```python
from build123d import *

# Parameters (mm, degrees)
SKETCH1_W           = 120
SKETCH1_H           = 90
BOSS_EXTRUDE1_DEPTH = 3
SKETCH2_W           = 4
SKETCH2_H           = 1.5
BOSS_EXTRUDE2_DEPTH = 15


with BuildPart() as part:
    # Sketch1 → Boss-Extrude1 (new body)
    with BuildSketch(Plane(origin=(0, 0, 0), x_dir=(0, 1, 0), z_dir=(0, 0, 1))):
        with Locations((-60, 45)):
            Rectangle(SKETCH1_W, SKETCH1_H)
    extrude(amount=BOSS_EXTRUDE1_DEPTH)

    # Sketch2 → Boss-Extrude2 (add)
    with BuildSketch(Plane.XY.offset(3)):
        with Locations((-88, -0.75)):
            Rectangle(SKETCH2_W, SKETCH2_H)
        with Locations((-60.6, -0.75)):
            Rectangle(SKETCH2_W, SKETCH2_H)
        with Locations((-29.4, -0.75)):
            Rectangle(SKETCH2_W, SKETCH2_H)
        with Locations((-2, -0.75)):
            Rectangle(SKETCH2_W, SKETCH2_H)
        with Locations((-88, -119.25)):
            Rectangle(SKETCH2_W, SKETCH2_H)
        with Locations((-60.6, -119.25)):
            Rectangle(SKETCH2_W, SKETCH2_H)
        with Locations((-29.4, -119.25)):
            Rectangle(SKETCH2_W, SKETCH2_H)
        with Locations((-2, -119.25)):
            Rectangle(SKETCH2_W, SKETCH2_H)
    extrude(amount=BOSS_EXTRUDE2_DEPTH)


solid = part.part
```
The listing builds one solid part. Answer for the finished solid, in the listing's coordinates (mm). A direction names the side the tool comes from. Give positions to 0.01 mm unless a question says otherwise; leave off trailing zeros. Write each loop counter-clockwise with the first axis right and the second up, starting at its lowest first coordinate (ties: lowest second). Pieces come first, ordered by that corner, then holes. Notation, with made-up numbers: (-9, 83.5) -> (10, 83.5) arc R5 cw to (10, 89.5) -> close; hole circle Ø2 at (51, -38.75). An arc over 180 degrees is marked (long way). Write item = value, one per line. Start each with the question number.
1) This flat-tipped pin is pushed along its axis until it touches: pin 1 (1 mm diameter, centred on x = -52, y = -87, fed in from +Z). Where does it stop, or does it pass through?
2) Which of the six approach directions +Z, -Z, +X, -X, +Y, -Y give full straight-line access (tool end or side, diameter ignored) to faces 1 (the face through (-45, 0, 1)), 2 (the face through (-61, -118.5, 10))?
3) The part is cut by section A-A, the plane z = 14.25. Count the separate pieces of the cut face and the enclosed holes in it, and give its area (3 significant figures).
4) The part is cut by section C-C, the plane x = -79.5. Determine the outline of the cut face in (y, z).
5) The part is cut by section B-B, the plane y = -36.5. Determine the outline of the cut face in (x, z).
6) Determine the mould class of faces 3 (the face through (-88, -1.5, 10)), 4 (the face through (0, -60, 2)), 5 (the face through (-45, -120, 1)) for opening direction Y: +Y half, -Y half, draft (parallel to the pull), parting line (faces both ways), or undercut.
7) Straight lines are drawn through the part: line 1 along Y through (x, z) = (-28, 10.75); line 2 along Z through (x, y) = (-56.5, -90). For each, find the intervals that lie inside material, in ascending order.
Solutions:
q1.pin_1 = 3
q2.face_1 = +Z, -Z, +X, -X, +Y
q2.face_2 = +Z, +X, -X
q3.separate_pieces = 8
q3.enclosed_holes = 0
q3.area = 48.0 mm²
q4.outline = (-120, 0) -> (0, 0) -> (0, 3) -> (-120, 3) -> close
q5.outline = (-90, 0) -> (0, 0) -> (0, 3) -> (-90, 3) -> close
q6.face_3 = undercut
q6.face_4 = draft
q6.face_5 = -Y half
q7.line_1 = -120 to -118.5, -1.5 to 0
q7.line_2 = 0 to 3
